For this review, take the finished solid that the model builds, in its own axes (mm). A direction names the side the tool comes from. Give positions to 0.01 mm unless a question says otherwise; leave off trailing zeros. Write each loop counter-clockwise with the first axis right and the second up, starting at its lowest first coordinate (ties: lowest second). Pieces come first, ordered by that corner, then holes.
Q1. Machinability: for faces 4 (the flat face through (7.72, 5.97, -2.46)), 5 (the flat face through (9, 2.5, -7)), 6 (the flat face through (13, 1, 2.647)), 7 (the flat face through (0.5, 1.2, 7.147)), 8 (the flat face through (0.773, 6.002, -2.465)), which of the approach directions +Z, -Z, +X, -X, +Y, -Y give a long, thin tool a straight path to every point of the face, cutting with its end or side? Answer none if there is none.
Q2. We need section B-B (z = -6). Write out the cut boundary in (x, y).
Q3. Mouldability with a two-part tool opening along Z and no side actions: class faces 1 (the flat face through (13, 1, -7.647)), 2 (the flat face through (13.374, 5.973, -2.465)), 3 (the flat face through (1, 1, 6)) as released by +Z, released by -Z, zero draft, split by the parting line, or undercut.
Q4. We need section C-C (x = 39). Write out the cut boundary in (y, z), then the cut area to 3 significant figures.
Q5. Insertion check: P1, Ø1, axis at x = 27.5, y = 1.5, coming from the -Z side; P2, Ø2, axis at x = 13.5, y = 1.5, coming from the -Z side; P3, Ø5, axis at x = 44, z = 1.5, coming from the -Y side. Each pin has a flat end and moves straight along its axis. Give the tip position at first contact, or say it passes through.
Q6. We need section A-A (y = 3.5). Write out the cut boundary in (x, z), then the cut area to 3 significant figures.
Q7. For line 1 (Z direction, x = 6.5, y = 2); line 2 (Z direction, x = 26, y = 6); line 3 (Y direction, x = 4, z = -2.25), list the stretches that pass through material, from the lowest coordinate up.
```python
from build123d import *

# Parameters (mm, degrees)
BLANKSKE_W          = 23.757
BLANKSKE_H          = 7
BLANK_DEPTH         = 5
TOOTHCUTSIM_DEPTH   = 26.26648074
TEETHCUTS_COUNT     = 9
TEETHCUTS_PITCH     = 2.827433385
SKETCH1_R           = 2.5
BOSS_EXTRUDE1_DEPTH = 32
SKETCH2_W           = 2.647496805
SKETCH2_H           = 2.5
BOSS_EXTRUDE2_DEPTH = 23.757
SKETCH3_W           = 5
SKETCH3_H           = 7
BOSS_EXTRUDE3_DEPTH = 3
SKETCH4_W           = 3
SKETCH4_H           = 2.5
BOSS_EXTRUDE4_DEPTH = 7
SKETCH5_W           = 2
SKETCH5_H           = 2.5
CUT_EXTRUDE1_DEPTH  = 1


with BuildPart() as part:
    # BlankSke → Blank (new body)
    with BuildSketch(Plane.XY):
        with Locations((11.8785, 3.5)):
            Rectangle(BLANKSKE_W, BLANKSKE_H)
    extrude(amount=-BLANK_DEPTH)

    # TooCutSkeSim → ToothCutSim (cut, through all)
    with BuildSketch(Plane.XY):
        Polygon((0.399391833, 4.975), (-0.399391833, 4.975), (-1.145676401, 7.0254), (1.145676401, 7.0254), align=None)
    toothcutsim = extrude(amount=-TOOTHCUTSIM_DEPTH, mode=Mode.SUBTRACT)

    # TeethCuts: ToothCutSim ×9
    with Locations(*[(i * TEETHCUTS_PITCH, 0, 0) for i in range(1, TEETHCUTS_COUNT)]):
        add(toothcutsim, mode=Mode.SUBTRACT)

    # Sketch1 → Boss-Extrude1 (add)
    with BuildSketch(Plane(origin=(23.757, 0, 0), x_dir=(0, 0, -1), z_dir=(1, 0, 0))):
        with Locations((2.5, 2.4875)):
            Circle(SKETCH1_R)
    extrude(amount=BOSS_EXTRUDE1_DEPTH)

    # Sketch2 → Boss-Extrude2 (add)
    with BuildSketch(Plane.ZY):
        with Locations((-6.323748402, 1.25)):
            Rectangle(SKETCH2_W, SKETCH2_H)
        with Locations((1.323748403, 1.25)):
            Rectangle(SKETCH2_W, SKETCH2_H)
    extrude(amount=-BOSS_EXTRUDE2_DEPTH)

    # Sketch3 → Boss-Extrude3 (add)
    with BuildSketch(Plane(origin=(23.757, 0, 0), x_dir=(0, 0, -1), z_dir=(1, 0, 0))):
        with Locations((2.5, 3.5)):
            Rectangle(SKETCH3_W, SKETCH3_H)
    extrude(amount=BOSS_EXTRUDE3_DEPTH)

    # Sketch4 → Boss-Extrude4 (add)
    with BuildSketch(Plane(origin=(0, 0, -7.647496805), x_dir=(-1, 0, 0), z_dir=(0, 0, -1))):
        with Locations((-1.5, 1.25)):
            Rectangle(SKETCH4_W, SKETCH4_H)
    boss_extrude4 = extrude(amount=BOSS_EXTRUDE4_DEPTH)

    # Mirror1: Boss-Extrude4 across plane
    add(boss_extrude4.mirror(Plane(origin=(0, 0, -2.5), x_dir=(1, 0, 0), z_dir=(0, 0, -1))))

    # Sketch5 → Cut-Extrude1 (cut)
    with BuildSketch(Plane.ZY):
        with Locations((-11.147496805, 1.25)):
            Rectangle(SKETCH5_W, SKETCH5_H)
    cut_extrude1 = extrude(amount=-CUT_EXTRUDE1_DEPTH, mode=Mode.SUBTRACT)

    # Mirror2: Cut-Extrude1 across plane
    add(cut_extrude1.mirror(Plane(origin=(0, 0, -2.5), x_dir=(1, 0, 0), z_dir=(0, 0, -1))), mode=Mode.SUBTRACT)


solid = part.part
```
Computed:
1. face 4: +Z, -Z, +Y
1. face 5: -Z, +X, -X, +Y
1. face 6: +Z, +X, +Y, -Y
1. face 7: -X, +Y, -Y
1. face 8: +Z, -Z, -X, +Y
2. outline: (0, 0) - (23.76, 0) - (23.76, 2.5) - (0, 2.5) - close
3. face 1: released by -Z
3. face 2: zero draft
3. face 3: undercut
4. outline: circle Ø5 at (2.49, -2.5)
4. area: 19.6 mm2
5. P1: stops at z = -4.95
5. P2: stops at z = -7.65
5. P3: stops at y = 0.49
6. outline: (0, -5) - (26.76, -5) - (26.76, -4.79) - (55.76, -4.79) - (55.76, -0.21) - (26.76, -0.21) - (26.76, 0) - (0, 0) - close
6. area: 266 mm2
7. line 1: z = -7.65 to 2.65
7. line 2: z = -5 to 0
7. line 3: y = 0 to 7
